Build history of the part. All positions in model axes, mm. Face numbers are marked on the shaded views. A direction names the side the tool comes from. Round coordinates to 2 decimals unless told otherwise and drop trailing zeros. Loops run counter-clockwise (first coordinate to the right, second up) from the corner with the lowest first, then second, coordinate; pieces in that order, holes last. Notation, with made-up numbers: M 44,-6 L 59,-6 A20 cw 59,29 Z; hole C 38,44 d1. An arc over 180 degrees is marked long. One line per item, written item: value.
```python
from build123d import *

# Parameters (mm, degrees)
SKETCH_1_R           = 1
EXTRUDE_1_DEPTH      = 2
SKETCH_2_R           = 5.65
EXTRUDE_2_DEPTH      = 2
EXTRUDE_3_DEPTH      = 5.5
EXTRUDE_3_DEPTH_BACK = 15
SKETCH_3_R           = 1.5
SKETCH_4_W           = 11.8
SKETCH_4_H           = 8
FILLET_1_R           = 1
SKETCH_5_OUTSIDE_W   = 53.038
SKETCH_5_OUTSIDE_H   = 55.038
CUT_EXTRUDE_4_DEPTH  = 1
FILLET_2_R           = 2
CHAMFER_1_SIZE       = 0.2
SKETCH_6_W           = 13
SKETCH_6_H           = 4
EXTRUDE_4_DEPTH      = 9


with BuildPart() as part:
    # 草图1 → 凸台-拉伸1 (new body)
    with BuildSketch(Plane(origin=(0, 0, 0), x_dir=(1, 0, 0), z_dir=(0, 1, 0))):
        with BuildLine():
            Line((-19.5, 15.975), (-13.13021325, 15.975))
            ThreePointArc((-13.13021325, 15.975), (0, 25.025), (13.13021325, 15.975))
            Line((13.13021325, 15.975), (19.5, 15.975))
            Line((19.5, 15.975), (19.5, -11.475))
            Line((19.5, -11.475), (15.5, -11.475))
            ThreePointArc((15.5, -11.475), (12.318019485, -12.793019485), (11, -15.975))
            Line((11, -15.975), (-11, -15.975))
            ThreePointArc((-11, -15.975), (-12.318019485, -12.793019485), (-15.5, -11.475))
            Line((-15.5, -11.475), (-19.5, -11.475))
            Line((-19.5, -11.475), (-19.5, 15.975))
        make_face()
        with Locations(Location((16, 10.975, 0), (0, 0, 270))):
            Circle(SKETCH_1_R, mode=Mode.SUBTRACT)
        with Locations(Location((-16, 10.975, 0), (0, 0, 90))):
            Circle(SKETCH_1_R, mode=Mode.SUBTRACT)
    extrude(amount=EXTRUDE_1_DEPTH)

    # 草图2 → 凸台-拉伸2 (add)
    with BuildSketch(Plane(origin=(0, 2, 0), x_dir=(1, 0, 0), z_dir=(0, 1, 0))):
        with Locations(Location((0, 10.975, 0), (0, 0, 90))):
            Circle(SKETCH_2_R)
    extrude(amount=EXTRUDE_2_DEPTH)

    # 草图3 → 凸台-拉伸3 (add, two sides: drawn at the far end of the back side and taken through both)
    with BuildSketch(Plane(origin=(0, 4, 0), x_dir=(1, 0, 0), z_dir=(0, 1, 0)).offset(-EXTRUDE_3_DEPTH_BACK)):
        with Locations(Location((0, 10.975, 0), (0, 0, 270))):
            Circle(SKETCH_3_R)
    extrude(amount=EXTRUDE_3_DEPTH + EXTRUDE_3_DEPTH_BACK)

    # 草图4 → 旋转1 (revolve)
    with BuildSketch(Plane(origin=(0, 0, 0), x_dir=(0, 0, -1), z_dir=(1, 0, 0))):
        with Locations((5.075, -7)):
            Rectangle(SKETCH_4_W, SKETCH_4_H)
    revolve(axis=Axis((0, 9.5, -10.975), (0, -1, 0)))

    # 圆角1
    fillet_1_edges = [part.edges().sort_by_distance(p)[0] for p in [
        (0, -11, -22.775),
    ]]
    fillet(fillet_1_edges, radius=FILLET_1_R)

    # 草图5 outside → 切除-拉伸4 (cut)
    with BuildSketch(Plane(origin=(0, 2, 0), x_dir=(1, 0, 0), z_dir=(0, 1, 0))):
        with Locations((0, 4.525)):
            Rectangle(SKETCH_5_OUTSIDE_W, SKETCH_5_OUTSIDE_H)
        with BuildLine():
            Line((-11, -8.975), (11, -8.975))
            Line((11, -8.975), (11, 6.975))
            Line((11, 6.975), (16, 6.975))
            ThreePointArc((16, 6.975), (20, 10.975), (16, 14.975))
            Line((16, 14.975), (13.468574535, 14.975))
            ThreePointArc((13.468574535, 14.975), (0, 25.025), (-13.468574535, 14.975))
            Line((-13.468574535, 14.975), (-16, 14.975))
            ThreePointArc((-16, 14.975), (-20, 10.975), (-16, 6.975))
            Line((-16, 6.975), (-11, 6.975))
            Line((-11, 6.975), (-11, -8.975))
        make_face(mode=Mode.SUBTRACT)
    extrude(amount=-CUT_EXTRUDE_4_DEPTH, mode=Mode.SUBTRACT)

    # 圆角2
    fillet_2_edges = [part.edges().sort_by_distance(p)[0] for p in [
        (-11, 1.5, -6.975),
        (11, 1.5, -6.975),
    ]]
    fillet(fillet_2_edges, radius=FILLET_2_R)

    # 倒角1
    chamfer_1_edges = [part.edges().sort_by_distance(p)[0] for p in [
        (0, 9.5, -12.475),
        (0, -3, -22.775),
    ]]
    chamfer(chamfer_1_edges, length=CHAMFER_1_SIZE)

    # 草图6 → 凸台-拉伸4 (add)
    with BuildSketch(Plane.XZ):
        with Locations((0, 12.975)):
            Rectangle(SKETCH_6_W, SKETCH_6_H)
    extrude(amount=EXTRUDE_4_DEPTH)


solid = part.part
```
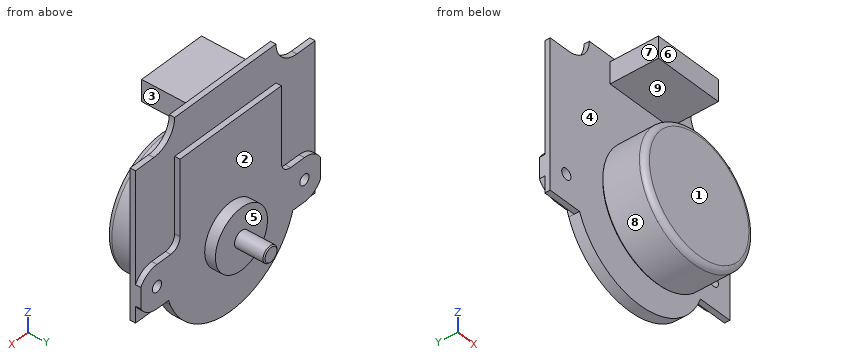
Item 1: Slice it at A-A, the plane y = -6.25. Give the cut face in (x, z) (3 decimals), and give its area (3 significant figures).
Check values:
outline: C 0,-10.975 d23.6; M -6.5,10.975 L 6.5,10.975 L 6.5,14.975 L -6.5,14.975 Z
area: 489 mm2
Item 2: Slice it at B-B, the plane z = 7. Give the cut face in (x, y).
Check values:
outline: M -19.5,0 L 19.5,0 L 19.5,1 L 11,1 L 11,2 L -11,2 L -11,1 L -19.5,1 Z
Item 3: Wall check: line 1 along Y through (x, z) = (-7, -7); line 2 along Z through (x, y) = (-16, 1.45) (3 decimals); line 3 along Z through (x, y) = (-16, 0.55) (3 decimals). Give the ranges that are in metal, low to high.
Check values:
line 1: y = -11 to -3, 0 to 2
line 2: z = -14.975 to -11.975, -9.975 to -6.975
line 3: z = -15.975 to -11.975, -9.975 to 11.475
Item 4: Which spindle directions (+Z, -Z, +X, -X, +Y, -Y) get a long thin tool onto all of the face, cutting with end or side? Do the marked faces 5, 6, 7, 8 and 9. Say none if no direction does.
Check values:
face 5: +Y
face 6: +Z, +X, -X, -Y
face 7: +Z, -X, -Y
face 8: -Y
face 9: +X, -X, -Y
Item 5: Pull direction Y, two halves, no side cores. Call the marked faces 1, 2, 3 and 4: pulls with the +Y half, pulls with the -Y half, needs draft (parallel to the pull), parting line crosses it, or undercut.
Check values:
face 1: pulls with the -Y half
face 2: pulls with the +Y half
face 3: needs draft
face 4: undercut
Item 6: Slice it at D-D, the plane y = 2.5. Give the cut face in (x, z) (3 decimals).
Check values:
outline: C 0,-10.975 d11.3
Item 7: Drop flat-ended pins along their axis: P1, Ø0.8, axis at x = 18.5, y = 0.5, coming from the +Z side (3 decimals); P2, Ø4.5, axis at y = -3.5, z = 13.5, coming from the -X side; P3, Ø0.8, axis at x = 14, y = 1.5, coming from the -Z side (3 decimals); P4, Ø4, axis at x = -7, y = 7, coming from the -Z side. Give the stop position or say it passes through.
Check values:
P1: stops at z = 11.475
P2: stops at x = -6.5
P3: stops at z = -14.975
P4: passes through
